```python
from build123d import *

# Parameters (mm, degrees)
F0_W     = 55
F0_H     = 560
F1_DEPTH = 800
F2_W     = 55
F2_H     = 560
F3_DEPTH = 25
F4_SIZE2 = 45
F4_SIZE  = 100
F5_W     = 746
F5_H     = 546
F6_DEPTH = 4
F8_DEPTH = 25


with BuildPart() as f1:
    # F0 (on Right) → F1 (new body)
    with BuildSketch(Plane.YZ):
        Polygon((22.5, 300), (-22.5, 300), (-22.5, -300), (22.5, -300), (22.5, -280), (22.5, 280), align=None)
        with Locations((50, 0)):
            Rectangle(F0_W, F0_H)
    extrude(amount=F1_DEPTH)

    # F2 (on face) + F0 (on Right) → F3 (cut, symmetric)
    with BuildSketch(Plane.YZ.offset(800)):
        with Locations((50, 0)):
            Rectangle(F2_W, F2_H)
    with BuildSketch(Plane.YZ):
        with Locations((50, 0)):
            Rectangle(F0_W, F0_H)
    extrude(amount=F3_DEPTH, both=True, mode=Mode.SUBTRACT)

    # F4
    f4_edges = [f1.edges().sort_by_distance(p)[0] for p in [
        (25, 77.5, 0),
        (400, 77.5, 280),
        (775, 77.5, 0),
        (400, 77.5, -280),
    ]]
    f4_side = f1.faces().sort_by_distance((400, 77.5, 0))[0]
    chamfer(f4_edges, length=F4_SIZE, length2=F4_SIZE2, reference=f4_side)

    # F5 (on face) → F6 (cut)
    with BuildSketch(Plane.XZ.offset(22.5)):
        with Locations((400, 0)):
            Rectangle(F5_W, F5_H)
    extrude(amount=-F6_DEPTH, mode=Mode.SUBTRACT)

    # F7 (on face) → F8 (cut)
    with BuildSketch(Plane(origin=(0, 77.5, 0), x_dir=(-1, 0, 0), z_dir=(0, 1, 0))):
        with BuildLine():
            ThreePointArc((-525, 94), (-529, 90), (-525, 86))
            Line((-525, 86), (-525, 94))
        make_face()
        with BuildLine():
            Line((-525, 94), (-525, 86))
            ThreePointArc((-525, 86), (-522.1715728753, 87.1715728753), (-521, 90))
            ThreePointArc((-521, 90), (-522.1715728753, 92.8284271247), (-525, 94))
        make_face()
        with BuildLine():
            ThreePointArc((-525, -86), (-529, -90), (-525, -94))
            Line((-525, -94), (-525, -86))
        make_face()
        with BuildLine():
            Line((-525, -86), (-525, -94))
            ThreePointArc((-525, -94), (-522.1715728753, -92.8284271247), (-521, -90))
            ThreePointArc((-521, -90), (-522.1715728753, -87.1715728753), (-525, -86))
        make_face()
        with BuildLine():
            ThreePointArc((-275, -86), (-279, -90), (-275, -94))
            Line((-275, -94), (-275, -86))
        make_face()
        with BuildLine():
            Line((-275, -86), (-275, -94))
            ThreePointArc((-275, -94), (-272.1715728753, -92.8284271247), (-271, -90))
            ThreePointArc((-271, -90), (-272.1715728753, -87.1715728753), (-275, -86))
        make_face()
        with BuildLine():
            ThreePointArc((-275, 94), (-279, 90), (-275, 86))
            Line((-275, 86), (-275, 94))
        make_face()
        with BuildLine():
            Line((-275, 94), (-275, 86))
            ThreePointArc((-275, 86), (-272.1715728753, 87.1715728753), (-271, 90))
            ThreePointArc((-271, 90), (-272.1715728753, 92.8284271247), (-275, 94))
        make_face()
    extrude(amount=-F8_DEPTH, mode=Mode.SUBTRACT)


solid = f1.part
```
Check sheet for the modelled part. Datum: model origin and axes. Units: mm. A direction names the side the tool comes from. Round coordinates to 2 decimals unless told otherwise and drop trailing zeros. Order: outer loops, then holes, each group sorted by start corner. A loop starts at its lowest first (then second) coordinate and runs counter-clockwise, first axis right, second up.
1) Section check A-A (x = 651). Record the boundary of the cut face in (y, z).
2) Tool access check on faces 4 (the flat face through (74.3, 54.685, -3.92)), 5 (the flat face through (398, 22.5, -290)). Record the directions out of +Z, -Z, +X, -X, +Y, -Y that give a thin tool (end or side, any length) a straight path to the whole face; none if there is none.
3) Scan lines: line 1 (Z direction, x = 524, y = 68.5); line 2 (Y direction, x = 367.5, z = 177.5); line 3 (X direction, y = 30, z = 234). Record each from-to range of solid material in increasing order.
4) Mould release check, pull along Z, two halves, no side actions. Record for faces 1 (the flat face through (395, -18.5, 4)), 2 (the flat face through (394, 0, 300)), 3 (the flat face through (396, 77.5, -3)): +Z half, -Z half, draft (parallel to the pull), parting line (faces both ways), or undercut.
5) Section check C-C (y = 42). Record the boundary of the cut face in (x, z), and give its area (3 significant figures).
6) Section check B-B (z = 106.5). Record the boundary of the cut face in (x, y), and give its area (3 significant figures).
7) Go/stop test with flat-tipped pins: pin 1 Ø9 at (x, z) = (277, -91) entering from +Y; pin 2 Ø11 at (y, z) = (28.5, -81) entering from +X; pin 3 Ø2.5 at (x, z) = (273.5, 91.5) entering from +Y; pin 4 Ø1 at (y, z) = (32, 16) entering from -X. Record where each tip stops, or that it passes through.
Result:
1. outline: (-22.5, -300) - (22.5, -300) - (22.5, -280) - (32.5, -280) - (77.5, -180) - (77.5, 180) - (32.5, 280) - (22.5, 280) - (22.5, 300) - (-22.5, 300) - (-22.5, 273) - (-18.5, 273) - (-18.5, -273) - (-22.5, -273) - close
2. face 4: +Z, -Z, -X, +Y
2. face 5: +Y
3. line 1: z = -200 to -93.87, -86.13 to 86.13, 93.87 to 200
3. line 2: y = -18.5 to 77.5
3. line 3: x = 25 to 775
4. face 1: undercut
4. face 2: +Z half
4. face 3: draft
5. outline: (46.11, -258.89) - (753.89, -258.89) - (753.89, 258.89) - (46.11, 258.89) - close
5. area: 366,000 mm2
6. outline: (0, -22.5) - (27, -22.5) - (27, -18.5) - (773, -18.5) - (773, -22.5) - (800, -22.5) - (800, 22.5) - (775, 22.5) - (775, 32.5) - (675, 77.5) - (125, 77.5) - (25, 32.5) - (25, 22.5) - (0, 22.5) - close
6. area: 69,800 mm2
7. pin 1: stops at y = 77.5
7. pin 2: stops at x = 775
7. pin 3: stops at y = 52.5
7. pin 4: stops at x = 25
